from build123d import *

# Parameters (mm, degrees)
SALIENTE_EXTRUIR1_DEPTH             = 7.95
CORTAR_EXTRUIR1_DEPTH               = 42.190806013
SALIENTE_EXTRUIR2_DEPTH             = 0.95
REDONDEO1_R                         = 2
CROQUIS5_W                          = 8.098391508
CROQUIS5_H                          = 3
SALIENTE_EXTRUIR3_DEPTH             = 1
REDONDEO2_R                         = 0.5
REDONDEO3_R                         = 1
SALIENTE_EXTRUIR5_DEPTH             = 16.075
SALIENTE_EXTRUIR6_START             = -2.8
SALIENTE_EXTRUIR6_DEPTH             = 3.2
REDONDEO4_R                         = 2
CORTAR_EXTRUIR2_REACH               = 48.175
CROQUIS9_R                          = 1.15
REDONDEO5_R                         = 0.2
CROQUIS10_R                         = 3.25
SALIENTE_EXTRUIR7_DEPTH             = 9
SALIENTE_EXTRUIR7_DIRECTION_2_REACH = 45.49
CORTAR_EXTRUIR3_DEPTH               = 3.2
REDONDEO6_R                         = 0.5
REDONDEO6_OF_SIMETR_A4_R            = 0.5
CORTAR_EXTRUIR4_REACH               = 47.21
CROQUIS12_R                         = 1.75
CROQUIS13_W                         = 41.090174937
CROQUIS13_H                         = 34.933198672
CORTAR_EXTRUIR6_DEPTH               = 33


with BuildPart() as part:
    # Croquis1 → Saliente-Extruir1 (new body)
    with BuildSketch(Plane(origin=(0, 0, 0), x_dir=(0, 0, -1), z_dir=(1, 0, 0))):
        Polygon((0, 0), (0, 12.2), (23.8, 12.2), (25.543157895, 15.8), (37.2, 15.8), (37.2, 13), (28.1, 13), (25.8, 8.25), (12.2, 8.25), (12.2, 0), align=None)
    extrude(amount=SALIENTE_EXTRUIR1_DEPTH)

    # Croquis2 → Cortar-Extruir1 (cut, through all)
    with BuildSketch(Plane(origin=(0, 15.8, 0), x_dir=(1, 0, 0), z_dir=(0, 1, 0))):
        with BuildLine():
            Line((0, 3.975), (0, -1.023351504))
            Line((0, -1.023351504), (7.95, -1.023351504))
            Line((7.95, -1.023351504), (7.95, 3.975))
            ThreePointArc((7.95, 3.975), (3.975, 0), (0, 3.975))
        make_face()
    extrude(amount=-CORTAR_EXTRUIR1_DEPTH, mode=Mode.SUBTRACT)

    # Croquis3 → Saliente-Extruir2 (add, symmetric)
    with BuildSketch(Plane.ZY.offset(-3.975)):
        Polygon((-23.8, 8.25), (-12.2, 1.25), (-12.2, 8.25), align=None)
    extrude(amount=SALIENTE_EXTRUIR2_DEPTH, both=True)

    # Redondeo1
    redondeo1_edges = [part.edges().sort_by_distance(p)[0] for p in [
        (0, 14.4, -37.2),
        (3.975, 15.8, -25.543157895),
        (3.975, 13, -28.1),
        (3.975, 8.25, -25.8),
        (7.95, 14.4, -37.2),
    ]]
    fillet(redondeo1_edges, radius=REDONDEO1_R)

    # Croquis5 → Saliente-Extruir3 (add, symmetric)
    with BuildSketch(Plane.ZY.offset(-3.975)):
        with Locations((-20.349195754, 11.935808548)):
            Rectangle(CROQUIS5_W, CROQUIS5_H)
    extrude(amount=SALIENTE_EXTRUIR3_DEPTH, both=True)

    # Redondeo2
    redondeo2_edges = [part.edges().sort_by_distance(p)[0] for p in [
        (3.975, 13.435808548, -16.3),
    ]]
    fillet(redondeo2_edges, radius=REDONDEO2_R)

    # Redondeo3
    redondeo3_edges = [part.edges().sort_by_distance(p)[0] for p in [
        (3.975, 0, -12.2),
    ]]
    fillet(redondeo3_edges, radius=REDONDEO3_R)

    # Croquis6 → Saliente-Extruir5 (add, symmetric)
    with BuildSketch(Plane(origin=(0, 6.1, 0), x_dir=(1, 0, 0), z_dir=(0, 1, 0))):
        with BuildLine():
            Line((2.775, 7.04908523), (2.775, 5.175))
            Line((2.775, 5.175), (0.90091477, 5.175))
            ThreePointArc((0.90091477, 5.175), (0.675, 3.975), (0.90091477, 2.775))
            Line((0.90091477, 2.775), (2.775, 2.775))
            Line((2.775, 2.775), (2.775, 0.90091477))
            ThreePointArc((2.775, 0.90091477), (3.975, 0.675), (5.175, 0.90091477))
            Line((5.175, 0.90091477), (5.175, 2.775))
            Line((5.175, 2.775), (7.04908523, 2.775))
            ThreePointArc((7.04908523, 2.775), (7.275, 3.975), (7.04908523, 5.175))
            Line((7.04908523, 5.175), (5.175, 5.175))
            Line((5.175, 5.175), (5.175, 7.04908523))
            ThreePointArc((5.175, 7.04908523), (3.975, 7.275), (2.775, 7.04908523))
        make_face()
    extrude(amount=SALIENTE_EXTRUIR5_DEPTH, both=True)

    # Croquis8 → Saliente-Extruir6 (add)
    with BuildSketch(Plane(origin=(0, 15.8, 0), x_dir=(1, 0, 0), z_dir=(0, 1, 0)).offset(SALIENTE_EXTRUIR6_START)):
        Polygon((3.975, 37.2), (5.95, 37.2), (7.95, 37.2), (7.95, 26.796861802), (3.975, 26.796861802), align=None)
    extrude(amount=SALIENTE_EXTRUIR6_DEPTH)

    # Redondeo4
    redondeo4_edges = [part.edges().sort_by_distance(p)[0] for p in [
        (7.95, 14.6, -37.2),
    ]]
    fillet(redondeo4_edges, radius=REDONDEO4_R)

    # Croquis9 → Cortar-Extruir2 (cut, up to next)
    with BuildSketch(Plane(origin=(0, 16.2, 0), x_dir=(1, 0, 0), z_dir=(0, 1, 0)), mode=Mode.PRIVATE) as cortar_extruir2_sk1:
        with Locations(Location((3.975, 33.45, 0), (0, 0, 270))):
            Circle(CROQUIS9_R)
    cortar_extruir2_tool1 = extrude(cortar_extruir2_sk1.sketch, amount=-CORTAR_EXTRUIR2_REACH, mode=Mode.PRIVATE) & part.part
    add(cortar_extruir2_tool1.solids().sort_by_distance((3.975, 16.2, -33.45))[0], mode=Mode.SUBTRACT)

    # Redondeo5
    redondeo5_edges = [part.edges().sort_by_distance(p)[0] for p in [
        (3.975, -9.975, -7.275),
        (0.675, -9.975, -3.975),
        (3.975, -9.975, -0.675),
        (7.275, -9.975, -3.975),
        (3.975, 22.175, -7.275),
        (0.675, 22.175, -3.975),
        (3.975, 22.175, -0.675),
        (7.275, 22.175, -3.975),
    ]]
    fillet(redondeo5_edges, radius=REDONDEO5_R)

    # Croquis10 → Saliente-Extruir7 (add)
    with BuildSketch(Plane(origin=(3.975, 0, 0), x_dir=(0, 0, -1), z_dir=(1, 0, 0))):
        with Locations((4.5, 6.1)):
            Circle(CROQUIS10_R)
    extrude(amount=SALIENTE_EXTRUIR7_DEPTH)

    # Saliente-Extruir7 direction 2: up to this face of the body (flat: up to its plane)
    saliente_extruir7_direction_2_end = Plane(part.part.faces().sort_by_distance((0, 8.735177915, -15.168906587))[0])
    # Croquis10 → Saliente-Extruir7 direction 2 (add, up to the picked face)
    with BuildSketch(Plane(origin=(3.975, 0, 0), x_dir=(0, 0, -1), z_dir=(1, 0, 0)), mode=Mode.PRIVATE) as saliente_extruir7_direction_2_sk1:
        with Locations((4.5, 6.1)):
            Circle(CROQUIS10_R)
    saliente_extruir7_direction_2_tool1 = split(extrude(saliente_extruir7_direction_2_sk1.sketch, amount=-SALIENTE_EXTRUIR7_DIRECTION_2_REACH, mode=Mode.PRIVATE), bisect_by=saliente_extruir7_direction_2_end, keep=Keep.BOTH, mode=Mode.PRIVATE)
    add(saliente_extruir7_direction_2_tool1.solids().sort_by(Axis((3.975, 6.1, -4.5), (-1, 0, 0)))[0])

    # Croquis11 → Cortar-Extruir3 (cut)
    with BuildSketch(Plane.ZY):
        with BuildLine():
            Line((-10.4, 10.1), (-4.5, 10.1))
            Line((-4.5, 10.1), (-4.5, 9.35))
            ThreePointArc((-4.5, 9.35), (-7.75, 6.1), (-4.5, 2.85))
            Line((-4.5, 2.85), (-4.5, 1.8))
            Line((-4.5, 1.8), (-10.4, 1.8))
            Line((-10.4, 1.8), (-10.4, 10.1))
        make_face()
    cortar_extruir3 = extrude(amount=-CORTAR_EXTRUIR3_DEPTH, mode=Mode.SUBTRACT)

    # Redondeo6
    redondeo6_edges = [part.edges().sort_by_distance(p)[0] for p in [
        (1.6, 1.8, -10.4),
        (1.6, 10.1, -10.4),
        (1.6, 10.1, -4.5),
        (1.6, 1.8, -4.5),
    ]]
    fillet(redondeo6_edges, radius=REDONDEO6_R)

    # Simetría4: Cortar-Extruir3 across plane
    add(cortar_extruir3.mirror(Plane(origin=(3.975, 0, 0), x_dir=(0, 0, 1), z_dir=(1, 0, 0))), mode=Mode.SUBTRACT)

    # Redondeo6 of Simetría4
    redondeo6_of_simetr_a4_edges = [part.edges().sort_by_distance(p)[0] for p in [
        (6.35, 1.8, -10.4),
        (6.35, 10.1, -10.4),
        (6.35, 10.1, -4.5),
        (6.35, 1.8, -4.5),
    ]]
    fillet(redondeo6_of_simetr_a4_edges, radius=REDONDEO6_OF_SIMETR_A4_R)

    # Croquis12 → Cortar-Extruir4 (cut, up to next)
    with BuildSketch(Plane(origin=(12.975, 0, 0), x_dir=(0, 0, -1), z_dir=(1, 0, 0)), mode=Mode.PRIVATE) as cortar_extruir4_sk1:
        with Locations((4.5, 6.1)):
            Circle(CROQUIS12_R)
    cortar_extruir4_tool1 = extrude(cortar_extruir4_sk1.sketch, amount=-CORTAR_EXTRUIR4_REACH, mode=Mode.PRIVATE) & part.part
    add(cortar_extruir4_tool1.solids().sort_by_distance((12.975, 6.1, -4.5))[0], mode=Mode.SUBTRACT)


with BuildPart() as body_2:
    # Simetría6: mirrored copy
    add(part.part.mirror(Plane.ZY.offset(10)))

    # Croquis13 → Cortar-Extruir6 (cut)
    with BuildSketch(Plane(origin=(-10, 0, 0), x_dir=(0, 0, -1), z_dir=(1, 0, 0))):
        with Locations((19.577078705, 6.209166246)):
            Rectangle(CROQUIS13_W, CROQUIS13_H)
    extrude(amount=-CORTAR_EXTRUIR6_DEPTH, mode=Mode.SUBTRACT)


solid = part.part
Check sheet for the modelled part. Datum: model origin and axes. Units: mm. A direction names the side the tool comes from. Round coordinates to 2 decimals unless told otherwise and drop trailing zeros. Order: outer loops, then holes, each group sorted by start corner. A loop starts at its lowest first (then second) coordinate and runs counter-clockwise, first axis right, second up.
Q1. Cross-section at C-C, the plane y = -6. Enter the section's corners in (x, z) (3 decimals).
Filled sheet:
outline: (0.901, -5.175) - (2.775, -5.175) - (2.775, -7.049) arc R3.3 ccw to (5.175, -7.049) - (5.175, -5.175) - (7.049, -5.175) arc R3.3 ccw to (7.049, -2.775) - (5.175, -2.775) - (5.175, -0.901) arc R3.3 ccw to (2.775, -0.901) - (2.775, -2.775) - (0.901, -2.775) arc R3.3 ccw to start
Q2. Scan lines: L1, parallel to X at y = 14.95, z = -33.45 (3 decimals); L2, parallel to Y at x = 3.5, z = -4.5 (3 decimals); L3, parallel to Y at x = 5.5, z = -15. Record each from-to range of solid material in increasing order.
Filled sheet:
L1: x = 0 to 2.825, 5.125 to 7.95
L2: y = -9.975 to 4.35, 7.85 to 22.175
L3: y = 8.25 to 12.2
Q3. Draft check along Z on faces 4 (the face through (2, 5, -12.2)), 5 (the face through (2, 1.8, -7)), 6 (the face through (4.925, 6, -16)). Enter one of: pulls with the +Z half, pulls with the -Z half, needs draft (parallel to the pull), parting line crosses it, or undercut.
Filled sheet:
face 4: pulls with the -Z half
face 5: undercut
face 6: needs draft
Q4. Depth check by flat-ended pin: P1, Ø0.6, axis at y = 16.5, z = -1.5, coming from the -X side (3 decimals); P2, Ø1.4, axis at y = 13, z = -20.5, coming from the +X side (3 decimals); P3, Ø12, axis at y = 18, z = -32, coming from the +X side. Enter the tip coordinate at first touch or a pass-through.
Filled sheet:
P1: stops at x = 2.775
P2: stops at x = 4.975
P3: stops at x = 7.95
Q5. Cross-section at B-B, the plane y = 5.5. Enter the section's corners in (x, z) (3 decimals).
Filled sheet:
outline: (0, -12.2) - (3.025, -12.2) - (3.025, -19.243) - (4.925, -19.243) - (4.925, -12.2) - (7.95, -12.2) - (7.95, -10.4) - (4.75, -10.4) - (4.75, -7.694) - (12.975, -7.694) - (12.975, -6.144) - (0, -6.144) - (0, -7.694) - (3.2, -7.694) - (3.2, -10.4) - (0, -10.4) - close; (0, -2.856) - (12.975, -2.856) - (12.975, -1.306) - (6.921, -1.306) arc R3.975 ccw to (1.029, -1.306) - (0, -1.306) - close
Q6. Cross-section at A-A, the plane z = -33.45. Enter the section's corners in (x, y) (3 decimals), plus the area to 4 significant figures.
Filled sheet:
outline: (0, 13) - (2.825, 13) - (2.825, 15.8) - (0, 15.8) - close; (5.125, 13) - (7.95, 13) - (7.95, 16.2) - (5.125, 16.2) - close
area: 16.95 mm2
Q7. Set-up check for faces 1 (the face through (4, 0, -8)), 2 (the face through (5.175, -5, -6)), 3 (the face through (4.75, 6, -8)): record each of +Z, -Z, +X, -X, +Y, -Y from which the full face is reachable in a straight line by a thin tool's end or side.
Filled sheet:
face 1: -Y
face 2: -Z, +X, -Y
face 3: +X
Q8. Cross-section at D-D, the plane x = 10.5. Enter the section's corners in (y, z), plus the area to 3 significant figures.
Filled sheet:
outline: circle Ø6.5 at (6.1, -4.5); hole circle Ø3.5 at (6.1, -4.5)
area: 23.6 mm2
